```python
from build123d import *

# Parameters (mm, degrees)
SKETCH1_W           = 42
SKETCH1_H           = 12
TAILLIGHTBASE_DEPTH = 2
SKETCH3_W           = 7
SKETCH3_H           = 12
MOUNTINGTABS_DEPTH  = 2
SKETCH4_R           = 1.375
MOUNTINGHOLES_DEPTH = 2
SKETCH5_R           = 2
CUT_EXTRUDE1_DEPTH  = 10


with BuildPart() as part:
    # Sketch1 → tailLightBase (new body)
    with BuildSketch(Plane.XY):
        with Locations((21, 6)):
            Rectangle(SKETCH1_W, SKETCH1_H)
    extrude(amount=TAILLIGHTBASE_DEPTH)

    # Sketch3 → mountingTabs (add)
    with BuildSketch(Plane.XY.offset(2)):
        with Locations((-3.5, 6)):
            Rectangle(SKETCH3_W, SKETCH3_H)
        with Locations((45.5, 6)):
            Rectangle(SKETCH3_W, SKETCH3_H)
    extrude(amount=-MOUNTINGTABS_DEPTH)

    # Sketch4 → mountingHoles (cut)
    with BuildSketch(Plane.XY.offset(2)):
        with Locations((-3.5, 9)):
            Circle(SKETCH4_R)
        with Locations((45.5, 9)):
            Circle(SKETCH4_R)
        with Locations((-3.5, 3)):
            Circle(SKETCH4_R)
        with Locations((45.5, 3)):
            Circle(SKETCH4_R)
    extrude(amount=-MOUNTINGHOLES_DEPTH, mode=Mode.SUBTRACT)

    # Sketch5 → Cut-Extrude1 (cut)
    with BuildSketch(Plane.XY.offset(2)):
        with Locations((3, 9)):
            Circle(SKETCH5_R)
        with Locations((9, 9)):
            Circle(SKETCH5_R)
        with Locations((15, 9)):
            Circle(SKETCH5_R)
        with Locations((21, 9)):
            Circle(SKETCH5_R)
        with Locations((27, 9)):
            Circle(SKETCH5_R)
        with Locations((33, 9)):
            Circle(SKETCH5_R)
        with Locations((39, 9)):
            Circle(SKETCH5_R)
        with Locations((39, 3)):
            Circle(SKETCH5_R)
        with Locations((33, 3)):
            Circle(SKETCH5_R)
        with Locations((27, 3)):
            Circle(SKETCH5_R)
        with Locations((21, 3)):
            Circle(SKETCH5_R)
        with Locations((15, 3)):
            Circle(SKETCH5_R)
        with Locations((9, 3)):
            Circle(SKETCH5_R)
        with Locations((3, 3)):
            Circle(SKETCH5_R)
    extrude(amount=-CUT_EXTRUDE1_DEPTH, mode=Mode.SUBTRACT)


solid = part.part
```
CAD build for the part. Positions are in the model's coordinates, mm. Coordinates: 2 decimals unless noted, no trailing zeros. Write each loop counter-clockwise with the first axis right and the second up, starting at its lowest first coordinate (ties: lowest second). Pieces come first, ordered by that corner, then holes. Notation, with made-up numbers: (-25, 37) -> (-12, 37) arc R6 ccw to (-12, 43) -> close; hole circle Ø5 at (14.5, 62.25). An arc over 180 degrees is marked (long way). Return JSON: item names as keys, results as strings. Group by question number.
Q1. Cut at C-C, the plane x = 45.5. Give the cut face in (y, z) (3 decimals).
Q2. Cut at B-B, the plane z = 0.7. State how many separate pieces and enclosed holes the cut face has, then the cut area to 3 significant figures.
Q3. Pull direction X, two halves, no side cores. Call faces 1 (the face through (13.4, 1.8, 1)), 2 (the face through (21, 6, 2)), 3 (the face through (49, 6, 1)): released by +X, released by -X, zero draft, split by the parting line, or undercut.
Q4. Cut at A-A, the plane x = 21. Give the cut face in (y, z).
Q5. Drill centre lines: line 1 (Y direction, x = 9, z = 0.7); line 2 (Y direction, x = -3.5, z = 1.1) (3 decimals). Where is each one in solid material? Low to high.
Q6. Flat gauge pins, fed straight in: pin 1 (3.5 mm diameter, centred on x = 21, y = 3, fed in from -Z); pin 2 (1.5 mm diameter, centred on x = 37.5, y = 4.5, fed in from -Z). Where does each tip first touch, or does it go through?
Returned:
{
 "1": {"outline": "(0, 0) -> (1.625, 0) -> (1.625, 2) -> (0, 2) -> close; (4.375, 0) -> (7.625, 0) -> (7.625, 2) -> (4.375, 2) -> close; (10.375, 0) -> (12, 0) -> (12, 2) -> (10.375, 2) -> close"},
 "2": {"separate pieces": "1", "enclosed holes": "18", "area": "472 mm2"},
 "3": {"face 1": "undercut", "face 2": "zero draft", "face 3": "released by +X"},
 "4": {"outline": "(0, 0) -> (1, 0) -> (1, 2) -> (0, 2) -> close; (5, 0) -> (7, 0) -> (7, 2) -> (5, 2) -> close; (11, 0) -> (12, 0) -> (12, 2) -> (11, 2) -> close"},
 "5": {"line 1": "y = 0 to 1, 5 to 7, 11 to 12", "line 2": "y = 0 to 1.625, 4.375 to 7.625, 10.375 to 12"},
 "6": {"pin 1": "passes through", "pin 2": "stops at z = 0"}
}
